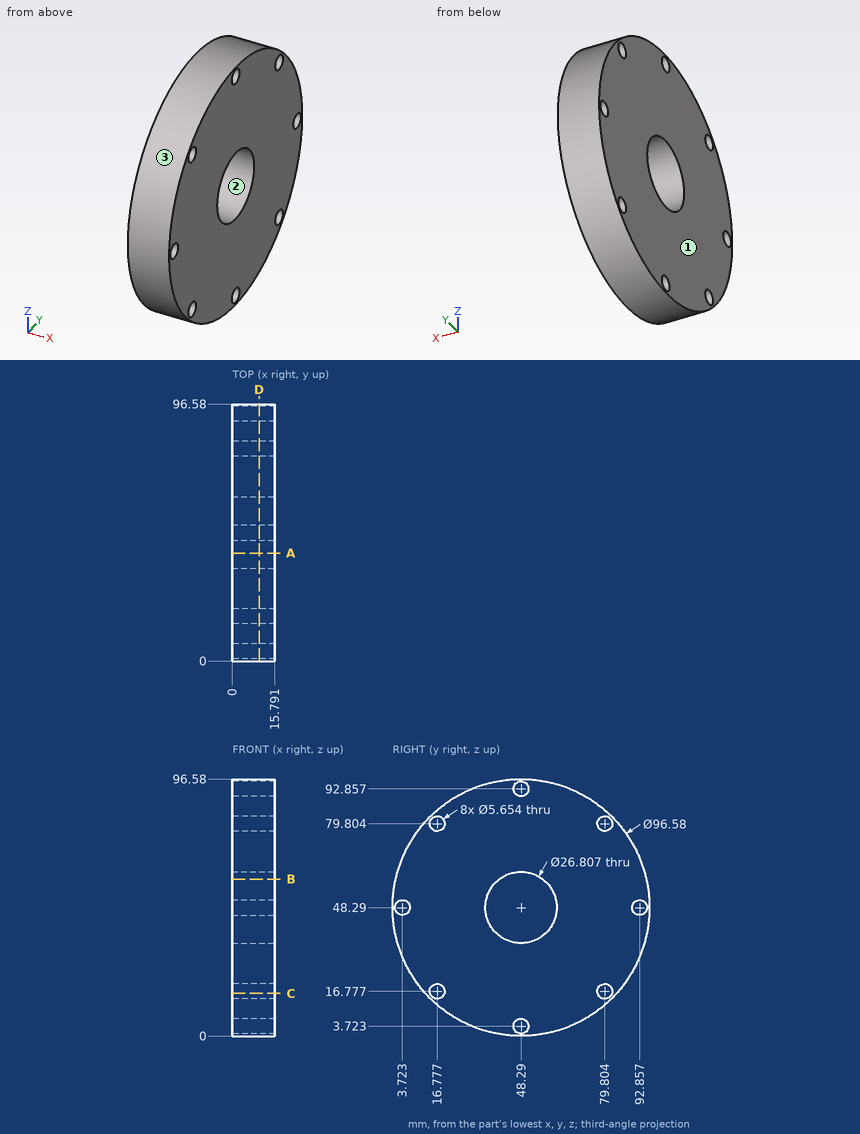
Check sheet for the drawn part. Datum: minimum x, y, z corner. Units: mm. Coordinates: 2 decimals unless noted, no trailing zeros. Loops run counter-clockwise (first coordinate to the right, second up) from the corner with the lowest first, then second, coordinate; pieces in that order, holes last. Notation, with made-up numbers: M 36,3 L 66,3 A17 ccw 66,19 Z; hole C 50,55.5 d2. An arc over 180 degrees is marked long. Answer as a JSON object with one key per item and string values.
1. Sectioned sample at D-D on x = 10. Count the separate pieces of the cut face and the enclosed holes in it, and give its area (3 significant figures).
Outcome:
{"separate pieces": "1", "enclosed holes": "9", "area": "6,560 mm²"}
2. Sectioned sample at A-A on y = 40.5. Record the cut outline in (x, z).
Outcome:
{"outline": "M 0,0.63 L 15.79,0.63 L 15.79,37.38 L 0,37.38 Z; M 0,59.2 L 15.79,59.2 L 15.79,95.95 L 0,95.95 Z"}
3. Scan lines: L1, parallel to Y at x = 2.75, z = 15.5 (1 decimal); L2, parallel to Y at x = 12, z = 15 (1 decimal); L3, parallel to Y at x = 13.5, z = 47.5 (1 decimal). Record each from-to range of solid material in increasing order. Write a range as from..to.
Outcome:
{"L1": "12.8..14.3, 19.3..77.3, 82.3..83.7", "L2": "13.3..14.6, 19..77.6, 82..83.3", "L3": "0..1, 6.4..34.9, 61.7..90.1, 95.6..96.6"}
4. Release check for a two-part mould opening along Y. For the marked faces 1, 2 and 3 record: pulls with the +Y half, pulls with the -Y half, needs draft (parallel to the pull), parting line crosses it, or undercut.
Outcome:
{"face 1": "needs draft", "face 2": "undercut", "face 3": "parting line crosses it"}
5. Depth check by flat-ended pin: P1, Ø3.5, axis at y = 48.29, z = 3.72, coming from the +X side; P2, Ø4, axis at x = 14, y = 52, coming from the +Z side; P3, Ø3, axis at x = 13, z = 43.5, coming from the -Y side. Enter the tip coordinate at first touch or a pass-through.
Outcome:
{"P1": "through", "P2": "z = 96.55", "P3": "y = 0.11"}
6. Sectioned sample at B-B on z = 59. Record the cut outline in (x, y), and give its area (3 significant figures).
Outcome:
{"outline": "M 0,1.2 L 15.79,1.2 L 15.79,40.23 L 0,40.23 Z; M 0,56.35 L 15.79,56.35 L 15.79,95.38 L 0,95.38 Z", "area": "1,230 mm²"}
7. Sectioned sample at C-C on z = 16. Record the cut outline in (x, y) (1 decimal), and give its area (3 significant figures).
Outcome:
{"outline": "M 0,12.4 L 15.8,12.4 L 15.8,14.1 L 0,14.1 Z; M 0,19.5 L 15.8,19.5 L 15.8,77.1 L 0,77.1 Z; M 0,82.5 L 15.8,82.5 L 15.8,84.2 L 0,84.2 Z", "area": "962 mm²"}
